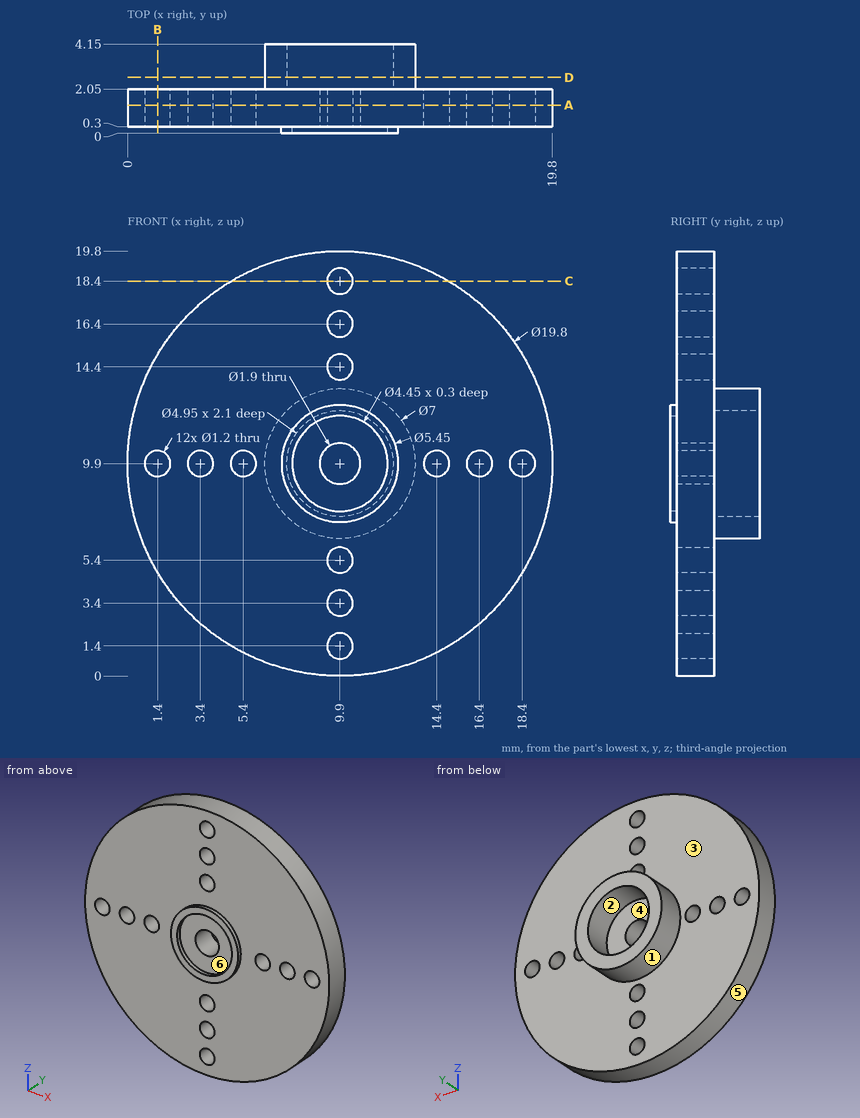
Print and shaded views of the part. All mm, measured from the part's lowest x, y and z. A direction names the side the tool comes from. Give positions to 0.01 mm unless a question says otherwise; leave off trailing zeros. Loops run counter-clockwise (first coordinate to the right, second up) from the corner with the lowest first, then second, coordinate; pieces in that order, holes last. Notation, with made-up numbers: (61.5, 65.5) -> (102.5, 65.5) arc R21 cw to (102.5, 86.5) -> close; hole circle Ø6 at (20.25, 48.25). An arc over 180 degrees is marked (long way). Answer in a Markdown table with one row per item.
Item 1: Slice it at A-A on y = 1.3. Give the number of separate pieces and of enclosed holes in the cut face, plus the area to 4 significant figures.
Findings below:
| item | result |
|---|---|
| separate pieces | 1 |
| enclosed holes | 13 |
| area | 291.5 mm² |
Item 2: Slice it at B-B on x = 1.4. Write the cut outline in (y, z), plus the area to 3 significant figures.
Findings below:
| item | result |
|---|---|
| outline | (0.3, 4.82) -> (2.05, 4.82) -> (2.05, 9.3) -> (0.3, 9.3) -> close; (0.3, 10.5) -> (2.05, 10.5) -> (2.05, 14.98) -> (0.3, 14.98) -> close |
| area | 15.7 mm² |
Item 3: Flat gauge pins, fed straight in: P1, Ø1.4, axis at x = 16.4, z = 9.9, coming from the -Y side; P2, Ø5, axis at x = 10.5, z = 17, coming from the +Y side. Where does each tip first touch, or does it go through?
Findings below:
| item | result |
|---|---|
| P1 | stops at y = 0.3 |
| P2 | stops at y = 2.05 |
Item 4: Tool access for the marked faces 4, 5 and 6: list every direction of +Z, -Z, +X, -X, +Y, -Y with a clear straight run to the whole face (end or side of a thin tool).
Findings below:
| item | result |
|---|---|
| face 4 | +Y |
| face 5 | +Y, -Y |
| face 6 | -Y |
Item 5: Slice it at C-C on z = 18.4. Write the cut outline in (x, y).
Findings below:
| item | result |
|---|---|
| outline | (4.82, 0.3) -> (9.3, 0.3) -> (9.3, 2.05) -> (4.82, 2.05) -> close; (10.5, 0.3) -> (14.98, 0.3) -> (14.98, 2.05) -> (10.5, 2.05) -> close |
Item 6: Probe line 1 along Y through (x, z) = (17.5, 12); line 2 along Z through (x, y) = (10.5, 3.55); line 3 along Z through (x, y) = (18.75, 0.65). List the from-to ranges inside material, lowest first. Write a range as [from, to].
Findings below:
| item | result |
|---|---|
| line 1 | y = [0.3, 2.05] |
| line 2 | z = [6.45, 7.5], [12.3, 13.35] |
| line 3 | z = [5.46, 9.41], [10.39, 14.34] |
Item 7: Mould opens along Z. For the marked faces 1, 2 and 3 say: pulls with the +Z half, pulls with the -Z half, needs draft (parallel to the pull), parting line crosses it, or undercut.
Findings below:
| item | result |
|---|---|
| face 1 | parting line crosses it |
| face 2 | undercut |
| face 3 | needs draft |
Item 8: Slice it at D-D on y = 2.6. Write the cut outline in (x, z) (3 decimals).
Findings below:
| item | result |
|---|---|
| outline | circle Ø7 at (9.9, 9.9); hole circle Ø4.95 at (9.9, 9.9) |
